Autodesk Inventor part; units mm, degrees
ref_plane "YZ Plane" through (0, 0, 0) normal (1, 0, 0) x (0, 1, 0)
ref_plane "XZ Plane" through (0, 0, 0) normal (0, 1, 0) x (-1, 0, 0)
ref_plane "XY Plane" through (0, 0, 0) normal (0, 0, 1) x (1, 0, 0)
sketch "Esquisse1" plane through (0, 0, 0) normal (0, 1, 0) x (-1, 0, 0)
  line L0 (0, 0) -> (0, 27) construction
  line L1 (0, 0) -> (24, 0) construction
  line L2 (24, 0) -> (24, 27) construction
  line L3 (24, 27) -> (0, 27) construction
  line L4 (0, 0) -> (8, 0) construction
  line L5 (8, 0) -> (16, 0) construction
  line L6 (16, 0) -> (24, 0) construction
  circle A0 centre (0, 0) radius 1
  circle A1 centre (8, 0) radius 1
  circle A2 centre (16, 0) radius 1
  circle A3 centre (24, 0) radius 1
  line L7 (24, 0) -> (29.5, 0) construction
  circle A4 centre (0, 27) radius 1
  circle A5 centre (8, 27) radius 1
  circle A6 centre (16, 27) radius 1
  circle A7 centre (24, 27) radius 1
  line L8 (29.5, 0) -> (29.5, 5.5) construction
  line L9 (29.5, 5.5) -> (29.5, 21.5) construction
  circle A8 centre (29.5, 21.5) radius 1
  circle A9 centre (29.5, 5.5) radius 1
  line L10 (0, 0) -> (0, -5) construction
  line L11 (0, -5) -> (-5, -5) construction
  line L12 (-5, -5) -> (-5, 32)
  line L13 (-5, 32) -> (35, 32)
  line L14 (35, 32) -> (35, -5)
  line L15 (35, -5) -> (-5, -5)
  line L16 (16, 0) -> (24, 0) construction
  dimension "d0" = 8
  dimension "d1" = 8
  dimension "d2" = 2
  dimension "d3" = 2
  dimension "d4" = 5.5
  dimension "d5" = 2
  dimension "d6" = 2
  dimension "d7" = 5.5
  dimension "d8" = 16
  dimension "d9" = 2
  dimension "d10" = 2
  dimension "d12" = 27
  dimension "d13" = 5
  dimension "d15" = 8
  dimension "d16" = 5.5
  dimension "d17" = 40
  dimension "d18" = 32
  dimension "d19" = 19
  dimension "d20" = 27
extrude "Extrusion1" add sketch "Esquisse1" along normal blind 2
properties part number "AX12_gabarit"
Build history of the part. All positions in model axes, mm. Coordinates: 2 decimals unless noted, no trailing zeros. Order: outer loops, then holes, each group sorted by start corner. A loop starts at its lowest first (then second) coordinate and runs counter-clockwise, first axis right, second up. Notation, with made-up numbers: (80, 39) - (114, 39) arc R25 ccw to (114, 70) - close; hole circle Ø7 at (70, 65). An arc over 180 degrees is marked (long way). Put each result on its own line as item: value.
1. Saw through at B-B (y = 0.45). Give the number of separate pieces and of enclosed holes in the cut face, and give its area (3 significant figures).
Answer sheet:
separate pieces: 1
enclosed holes: 10
area: 1,450 mm^2
2. Pull direction Z, two halves, no side cores. Call faces 1 (the face through (0, 1, 28)), 2 (the face through (-15, 1, 32)), 3 (the face through (-15, 1, -5)): pulls with the +Z half, pulls with the -Z half, needs draft (parallel to the pull), parting line crosses it, or undercut.
Answer sheet:
face 1: undercut
face 2: pulls with the +Z half
face 3: pulls with the -Z half
3. Saw through at D-D (x = -7.5). Write the cut outline in (y, z), and give its area (3 significant figures).
Answer sheet:
outline: (0, -5) - (2, -5) - (2, -0.87) - (0, -0.87) - close; (0, 0.87) - (2, 0.87) - (2, 26.13) - (0, 26.13) - close; (0, 27.87) - (2, 27.87) - (2, 32) - (0, 32) - close
area: 67.1 mm^2
4. Saw through at A-A (z = 21.5). Write the cut outline in (x, y).
Answer sheet:
outline: (-35, 0) - (-30.5, 0) - (-30.5, 2) - (-35, 2) - close; (-28.5, 0) - (5, 0) - (5, 2) - (-28.5, 2) - close
5. Saw through at C-C (x = -29.5). Write the cut outline in (y, z).
Answer sheet:
outline: (0, -5) - (2, -5) - (2, 4.5) - (0, 4.5) - close; (0, 6.5) - (2, 6.5) - (2, 20.5) - (0, 20.5) - close; (0, 22.5) - (2, 22.5) - (2, 32) - (0, 32) - close
6. Probe line 1 along Z through (x, y) = (-24, 1.8); line 2 along X through (y, z) = (0.85, 22). List the from-to ranges inside material, lowest first. Write a range as [from, to].
Answer sheet:
line 1: z = [-5, -1], [1, 26], [28, 32]
line 2: x = [-35, -30.37], [-28.63, 5]
7. Drop a flat-ended pin along its axis: P1, Ø1.8, axis at x = 0, z = 27, coming from the -Y side. Give the stop position or say it passes through.
Answer sheet:
P1: passes through
